```python
from build123d import *

# Parameters (mm, degrees)
SKETCH1_R           = 1.65
SKETCH1_R_2         = 10.1
BOSS_EXTRUDE1_DEPTH = 1.9
SKETCH2_W           = 1.9
SKETCH2_H           = 38
BOSS_EXTRUDE2_DEPTH = 44.5
CUT_EXTRUDE1_REACH  = 89.82
FILLET1_R           = 2


with BuildPart() as part:
    # Sketch1 → Boss-Extrude1 (new body)
    with BuildSketch(Plane(origin=(0, 0, 0), x_dir=(1, 0, 0), z_dir=(0, 1, 0))):
        with BuildLine():
            Line((-37, 19), (-37, -19))
            Line((-37, -19), (19, -19))
            ThreePointArc((19, -19), (31.785488519, -13.086252381), (37, -1.44e-07))
            ThreePointArc((37, -1.44e-07), (31.785488618, 13.086252276), (19, 19))
            Line((19, 19), (-37, 19))
        make_face()
        with Locations(Location((25.297222222, -12.687272165, 0), (0, 0, 90))):
            Circle(SKETCH1_R, mode=Mode.SUBTRACT)
        with BuildLine():
            ThreePointArc((-15.227777778, -3.8), (-19.027777778, 0), (-15.227777778, 3.8))
            Line((-15.227777778, 3.8), (-5.227777778, 3.8))
            ThreePointArc((-5.227777778, 3.8), (-1.427777778, 0), (-5.227777778, -3.8))
            Line((-5.227777778, -3.8), (-15.227777778, -3.8))
        make_face(mode=Mode.SUBTRACT)
        with Locations(Location((3.322222222, 0, 0), (0, 0, 90))):
            Circle(SKETCH1_R, mode=Mode.SUBTRACT)
        with Locations(Location((17.972222222, 0, 0), (0, 0, 90))):
            Circle(SKETCH1_R_2, mode=Mode.SUBTRACT)
        with Locations(Location((25.297222222, 12.687272165, 0), (0, 0, 90))):
            Circle(SKETCH1_R, mode=Mode.SUBTRACT)
    extrude(amount=BOSS_EXTRUDE1_DEPTH)

    # Sketch2 → Boss-Extrude2 (add)
    with BuildSketch(Plane(origin=(0, 1.9, 0), x_dir=(1, 0, 0), z_dir=(0, 1, 0))):
        with Locations((-36.05, 0)):
            Rectangle(SKETCH2_W, SKETCH2_H)
    extrude(amount=BOSS_EXTRUDE2_DEPTH)

    # Sketch3 → Cut-Extrude1 (cut, up to next)
    with BuildSketch(Plane(origin=(-35.1, 0, 0), x_dir=(0, 0, -1), z_dir=(1, 0, 0)), mode=Mode.PRIVATE) as cut_extrude1_sk1:
        with BuildLine():
            ThreePointArc((-9.4, 38.95), (-12.55, 42.1), (-15.7, 38.95))
            Line((-15.7, 38.95), (-9.4, 38.95))
        make_face()
    cut_extrude1_tool1 = extrude(cut_extrude1_sk1.sketch, amount=-CUT_EXTRUDE1_REACH, mode=Mode.PRIVATE) & part.part
    # Sketch3 → Cut-Extrude1 (cut, up to next)
    with BuildSketch(Plane(origin=(-35.1, 0, 0), x_dir=(0, 0, -1), z_dir=(1, 0, 0)), mode=Mode.PRIVATE) as cut_extrude1_sk2:
        with BuildLine():
            Line((-9.4, 38.95), (-15.7, 38.95))
            ThreePointArc((-15.7, 38.95), (-12.55, 35.8), (-9.4, 38.95))
        make_face()
    cut_extrude1_tool2 = extrude(cut_extrude1_sk2.sketch, amount=-CUT_EXTRUDE1_REACH, mode=Mode.PRIVATE) & part.part
    # Sketch3 → Cut-Extrude1 (cut, up to next)
    with BuildSketch(Plane(origin=(-35.1, 0, 0), x_dir=(0, 0, -1), z_dir=(1, 0, 0)), mode=Mode.PRIVATE) as cut_extrude1_sk3:
        with BuildLine():
            ThreePointArc((-9.4, 38.95), (-12.55, 42.1), (-15.7, 38.95))
            Line((-15.7, 38.95), (-9.4, 38.95))
        make_face()
    cut_extrude1_tool3 = extrude(cut_extrude1_sk3.sketch, amount=-CUT_EXTRUDE1_REACH, mode=Mode.PRIVATE) & part.part
    # Sketch3 → Cut-Extrude1 (cut, up to next)
    with BuildSketch(Plane(origin=(-35.1, 0, 0), x_dir=(0, 0, -1), z_dir=(1, 0, 0)), mode=Mode.PRIVATE) as cut_extrude1_sk4:
        with BuildLine():
            Line((-9.4, 38.95), (-15.7, 38.95))
            ThreePointArc((-15.7, 38.95), (-12.55, 35.8), (-9.4, 38.95))
        make_face()
    cut_extrude1_tool4 = extrude(cut_extrude1_sk4.sketch, amount=-CUT_EXTRUDE1_REACH, mode=Mode.PRIVATE) & part.part
    # Sketch3 → Cut-Extrude1 (cut, up to next)
    with BuildSketch(Plane(origin=(-35.1, 0, 0), x_dir=(0, 0, -1), z_dir=(1, 0, 0)), mode=Mode.PRIVATE) as cut_extrude1_sk5:
        with BuildLine():
            Line((-15.7, 38.95), (-15.7, 26.95))
            ThreePointArc((-15.7, 26.95), (-12.55, 30.1), (-9.4, 26.95))
            Line((-9.4, 26.95), (-9.4, 38.95))
            ThreePointArc((-9.4, 38.95), (-12.55, 35.8), (-15.7, 38.95))
        make_face()
    cut_extrude1_tool5 = extrude(cut_extrude1_sk5.sketch, amount=-CUT_EXTRUDE1_REACH, mode=Mode.PRIVATE) & part.part
    # Sketch3 → Cut-Extrude1 (cut, up to next)
    with BuildSketch(Plane(origin=(-35.1, 0, 0), x_dir=(0, 0, -1), z_dir=(1, 0, 0)), mode=Mode.PRIVATE) as cut_extrude1_sk6:
        with BuildLine():
            ThreePointArc((-9.4, 26.95), (-12.55, 30.1), (-15.7, 26.95))
            Line((-15.7, 26.95), (-9.4, 26.95))
        make_face()
    cut_extrude1_tool6 = extrude(cut_extrude1_sk6.sketch, amount=-CUT_EXTRUDE1_REACH, mode=Mode.PRIVATE) & part.part
    # Sketch3 → Cut-Extrude1 (cut, up to next)
    with BuildSketch(Plane(origin=(-35.1, 0, 0), x_dir=(0, 0, -1), z_dir=(1, 0, 0)), mode=Mode.PRIVATE) as cut_extrude1_sk7:
        with BuildLine():
            Line((-9.4, 26.95), (-15.7, 26.95))
            ThreePointArc((-15.7, 26.95), (-12.55, 23.8), (-9.4, 26.95))
        make_face()
    cut_extrude1_tool7 = extrude(cut_extrude1_sk7.sketch, amount=-CUT_EXTRUDE1_REACH, mode=Mode.PRIVATE) & part.part
    # Sketch3 → Cut-Extrude1 (cut, up to next)
    with BuildSketch(Plane(origin=(-35.1, 0, 0), x_dir=(0, 0, -1), z_dir=(1, 0, 0)), mode=Mode.PRIVATE) as cut_extrude1_sk8:
        with BuildLine():
            Line((9.4, 38.95), (9.4, 26.95))
            ThreePointArc((9.4, 26.95), (12.55, 30.1), (15.7, 26.95))
            Line((15.7, 26.95), (15.7, 38.95))
            ThreePointArc((15.7, 38.95), (12.55, 35.8), (9.4, 38.95))
        make_face()
    cut_extrude1_tool8 = extrude(cut_extrude1_sk8.sketch, amount=-CUT_EXTRUDE1_REACH, mode=Mode.PRIVATE) & part.part
    # Sketch3 → Cut-Extrude1 (cut, up to next)
    with BuildSketch(Plane(origin=(-35.1, 0, 0), x_dir=(0, 0, -1), z_dir=(1, 0, 0)), mode=Mode.PRIVATE) as cut_extrude1_sk9:
        with BuildLine():
            ThreePointArc((15.7, 38.95), (12.55, 42.1), (9.4, 38.95))
            Line((9.4, 38.95), (15.7, 38.95))
        make_face()
    cut_extrude1_tool9 = extrude(cut_extrude1_sk9.sketch, amount=-CUT_EXTRUDE1_REACH, mode=Mode.PRIVATE) & part.part
    # Sketch3 → Cut-Extrude1 (cut, up to next)
    with BuildSketch(Plane(origin=(-35.1, 0, 0), x_dir=(0, 0, -1), z_dir=(1, 0, 0)), mode=Mode.PRIVATE) as cut_extrude1_sk10:
        with BuildLine():
            Line((15.7, 38.95), (9.4, 38.95))
            ThreePointArc((9.4, 38.95), (12.55, 35.8), (15.7, 38.95))
        make_face()
    cut_extrude1_tool10 = extrude(cut_extrude1_sk10.sketch, amount=-CUT_EXTRUDE1_REACH, mode=Mode.PRIVATE) & part.part
    # Sketch3 → Cut-Extrude1 (cut, up to next)
    with BuildSketch(Plane(origin=(-35.1, 0, 0), x_dir=(0, 0, -1), z_dir=(1, 0, 0)), mode=Mode.PRIVATE) as cut_extrude1_sk11:
        with BuildLine():
            ThreePointArc((15.7, 38.95), (12.55, 42.1), (9.4, 38.95))
            Line((9.4, 38.95), (15.7, 38.95))
        make_face()
    cut_extrude1_tool11 = extrude(cut_extrude1_sk11.sketch, amount=-CUT_EXTRUDE1_REACH, mode=Mode.PRIVATE) & part.part
    # Sketch3 → Cut-Extrude1 (cut, up to next)
    with BuildSketch(Plane(origin=(-35.1, 0, 0), x_dir=(0, 0, -1), z_dir=(1, 0, 0)), mode=Mode.PRIVATE) as cut_extrude1_sk12:
        with BuildLine():
            Line((15.7, 38.95), (9.4, 38.95))
            ThreePointArc((9.4, 38.95), (12.55, 35.8), (15.7, 38.95))
        make_face()
    cut_extrude1_tool12 = extrude(cut_extrude1_sk12.sketch, amount=-CUT_EXTRUDE1_REACH, mode=Mode.PRIVATE) & part.part
    # Sketch3 → Cut-Extrude1 (cut, up to next)
    with BuildSketch(Plane(origin=(-35.1, 0, 0), x_dir=(0, 0, -1), z_dir=(1, 0, 0)), mode=Mode.PRIVATE) as cut_extrude1_sk13:
        with BuildLine():
            ThreePointArc((15.7, 26.95), (12.55, 30.1), (9.4, 26.95))
            Line((9.4, 26.95), (15.7, 26.95))
        make_face()
    cut_extrude1_tool13 = extrude(cut_extrude1_sk13.sketch, amount=-CUT_EXTRUDE1_REACH, mode=Mode.PRIVATE) & part.part
    # Sketch3 → Cut-Extrude1 (cut, up to next)
    with BuildSketch(Plane(origin=(-35.1, 0, 0), x_dir=(0, 0, -1), z_dir=(1, 0, 0)), mode=Mode.PRIVATE) as cut_extrude1_sk14:
        with BuildLine():
            Line((15.7, 26.95), (9.4, 26.95))
            ThreePointArc((9.4, 26.95), (12.55, 23.8), (15.7, 26.95))
        make_face()
    cut_extrude1_tool14 = extrude(cut_extrude1_sk14.sketch, amount=-CUT_EXTRUDE1_REACH, mode=Mode.PRIVATE) & part.part
    # Sketch3 → Cut-Extrude1 (cut, up to next)
    with BuildSketch(Plane(origin=(-35.1, 0, 0), x_dir=(0, 0, -1), z_dir=(1, 0, 0)), mode=Mode.PRIVATE) as cut_extrude1_sk15:
        with BuildLine():
            ThreePointArc((15.7, 26.95), (12.55, 30.1), (9.4, 26.95))
            Line((9.4, 26.95), (15.7, 26.95))
        make_face()
    cut_extrude1_tool15 = extrude(cut_extrude1_sk15.sketch, amount=-CUT_EXTRUDE1_REACH, mode=Mode.PRIVATE) & part.part
    # Sketch3 → Cut-Extrude1 (cut, up to next)
    with BuildSketch(Plane(origin=(-35.1, 0, 0), x_dir=(0, 0, -1), z_dir=(1, 0, 0)), mode=Mode.PRIVATE) as cut_extrude1_sk16:
        with BuildLine():
            Line((15.7, 26.95), (9.4, 26.95))
            ThreePointArc((9.4, 26.95), (12.55, 23.8), (15.7, 26.95))
        make_face()
    cut_extrude1_tool16 = extrude(cut_extrude1_sk16.sketch, amount=-CUT_EXTRUDE1_REACH, mode=Mode.PRIVATE) & part.part
    # Sketch3 → Cut-Extrude1 (cut, up to next)
    with BuildSketch(Plane(origin=(-35.1, 0, 0), x_dir=(0, 0, -1), z_dir=(1, 0, 0)), mode=Mode.PRIVATE) as cut_extrude1_sk17:
        with BuildLine():
            ThreePointArc((-9.4, 26.95), (-12.55, 30.1), (-15.7, 26.95))
            Line((-15.7, 26.95), (-9.4, 26.95))
        make_face()
    cut_extrude1_tool17 = extrude(cut_extrude1_sk17.sketch, amount=-CUT_EXTRUDE1_REACH, mode=Mode.PRIVATE) & part.part
    # Sketch3 → Cut-Extrude1 (cut, up to next)
    with BuildSketch(Plane(origin=(-35.1, 0, 0), x_dir=(0, 0, -1), z_dir=(1, 0, 0)), mode=Mode.PRIVATE) as cut_extrude1_sk18:
        with BuildLine():
            Line((-9.4, 26.95), (-15.7, 26.95))
            ThreePointArc((-15.7, 26.95), (-12.55, 23.8), (-9.4, 26.95))
        make_face()
    cut_extrude1_tool18 = extrude(cut_extrude1_sk18.sketch, amount=-CUT_EXTRUDE1_REACH, mode=Mode.PRIVATE) & part.part
    add(cut_extrude1_tool1.solids().sort_by_distance((-35.1, 40.286902, 12.55))[0], mode=Mode.SUBTRACT)
    add(cut_extrude1_tool2.solids().sort_by_distance((-35.1, 37.613098, 12.55))[0], mode=Mode.SUBTRACT)
    add(cut_extrude1_tool3.solids().sort_by_distance((-35.1, 40.286902, 12.55))[0], mode=Mode.SUBTRACT)
    add(cut_extrude1_tool4.solids().sort_by_distance((-35.1, 37.613098, 12.55))[0], mode=Mode.SUBTRACT)
    add(cut_extrude1_tool5.solids().sort_by_distance((-35.1, 32.95, 12.55))[0], mode=Mode.SUBTRACT)
    add(cut_extrude1_tool6.solids().sort_by_distance((-35.1, 28.286902, 12.55))[0], mode=Mode.SUBTRACT)
    add(cut_extrude1_tool7.solids().sort_by_distance((-35.1, 25.613098, 12.55))[0], mode=Mode.SUBTRACT)
    add(cut_extrude1_tool8.solids().sort_by_distance((-35.1, 32.95, -12.55))[0], mode=Mode.SUBTRACT)
    add(cut_extrude1_tool9.solids().sort_by_distance((-35.1, 40.286902, -12.55))[0], mode=Mode.SUBTRACT)
    add(cut_extrude1_tool10.solids().sort_by_distance((-35.1, 37.613098, -12.55))[0], mode=Mode.SUBTRACT)
    add(cut_extrude1_tool11.solids().sort_by_distance((-35.1, 40.286902, -12.55))[0], mode=Mode.SUBTRACT)
    add(cut_extrude1_tool12.solids().sort_by_distance((-35.1, 37.613098, -12.55))[0], mode=Mode.SUBTRACT)
    add(cut_extrude1_tool13.solids().sort_by_distance((-35.1, 28.286902, -12.55))[0], mode=Mode.SUBTRACT)
    add(cut_extrude1_tool14.solids().sort_by_distance((-35.1, 25.613098, -12.55))[0], mode=Mode.SUBTRACT)
    add(cut_extrude1_tool15.solids().sort_by_distance((-35.1, 28.286902, -12.55))[0], mode=Mode.SUBTRACT)
    add(cut_extrude1_tool16.solids().sort_by_distance((-35.1, 25.613098, -12.55))[0], mode=Mode.SUBTRACT)
    add(cut_extrude1_tool17.solids().sort_by_distance((-35.1, 28.286902, 12.55))[0], mode=Mode.SUBTRACT)
    add(cut_extrude1_tool18.solids().sort_by_distance((-35.1, 25.613098, 12.55))[0], mode=Mode.SUBTRACT)

    # Fillet1
    fillet1_edges = [part.edges().sort_by_distance(p)[0] for p in [
        (-37, 0, 0),
        (-35.1, 1.9, 0),
    ]]
    fillet(fillet1_edges, radius=FILLET1_R)


solid = part.part
```
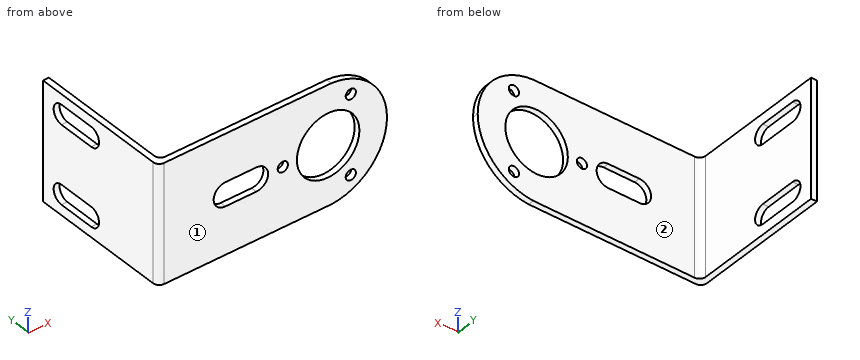
Part model, mm, in its own coordinate system. Face numbers are marked on the shaded views. A direction names the side the tool comes from. Coordinates: 2 decimals unless noted, no trailing zeros. Write each loop counter-clockwise with the first axis right and the second up, starting at its lowest first coordinate (ties: lowest second). Pieces come first, ordered by that corner, then holes.
Item 1: Slice it at B-B (z = -7.5). Write the cut outline in (x, y), and give its area (3 significant figures).
Item 2: Slice it at D-D (z = 13). Write the cut outline in (x, y), and give its area (3 significant figures).
Item 3: Which spindle directions (+Z, -Z, +X, -X, +Y, -Y) get a long thin tool onto all of the face, cutting with end or side? Do the marked faces 1 and 2. Say none if no direction does.
Item 4: Slice it at C-C (y = 33). Write the cut outline in (x, z).
Item 5: Pin check, flat tips, straight feed: pin 1 (10 mm diameter, centred on y = 38.5, z = -3.5, fed in from +X); pin 2 (11.5 mm diameter, centred on x = -14, z = 6, fed in from +Y). Stop position of each tip, or through.
Item 6: Probe line 1 (Y direction, x = 25, z = 16); line 2 (X direction, y = 12, z = -15). List the from-to ranges inside material, lowest first.
Item 7: Slice it at A-A (x = -12). Write the cut outline in (y, z), and give its area (3 significant figures).
Results found:
1. outline: (-37, 2) arc R2 ccw to (-35, 0) - (11.21, 0) - (11.21, 1.9) - (-33.1, 1.9) arc R2 cw to (-35.1, 3.9) - (-35.1, 46.4) - (-37, 46.4) - close; (24.74, 0) - (35.46, 0) - (35.46, 1.9) - (24.74, 1.9) - close
1. area: 197 mm2
2. outline: (-37, 2) arc R2 ccw to (-35, 0) - (23.68, 0) - (23.68, 1.9) - (-33.1, 1.9) arc R2 cw to (-35.1, 3.9) - (-35.1, 23.83) - (-37, 23.83) - close; (-37, 42.07) - (-35.1, 42.07) - (-35.1, 46.4) - (-37, 46.4) - close; (26.92, 0) - (31.87, 0) - (31.87, 1.9) - (26.92, 1.9) - close
2. area: 175 mm2
3. face 1: +Z, -Z, +X, -X, -Y
3. face 2: +Z, -Z, +X, +Y
4. outline: (-37, -19) - (-35.1, -19) - (-35.1, -15.7) - (-37, -15.7) - close; (-37, -9.4) - (-35.1, -9.4) - (-35.1, 9.4) - (-37, 9.4) - close; (-37, 15.7) - (-35.1, 15.7) - (-35.1, 19) - (-37, 19) - close
5. pin 1: stops at x = -35.1
5. pin 2: stops at y = 1.9
6. line 1: y = 0 to 1.9
6. line 2: x = -37 to -35.1
7. outline: (0, -19) - (1.9, -19) - (1.9, -3.8) - (0, -3.8) - close; (0, 3.8) - (1.9, 3.8) - (1.9, 19) - (0, 19) - close
7. area: 57.8 mm2
